Answer from the drawing. Dimensions are ordinates in mm from the lowest x, y and z of the part. A direction names the side the tool comes from. Give positions to 0.01 mm unless a question says otherwise; leave off trailing zeros. Order: outer loops, then holes, each group sorted by start corner. A loop starts at its lowest first (then second) coordinate and runs counter-clockwise, first axis right, second up.
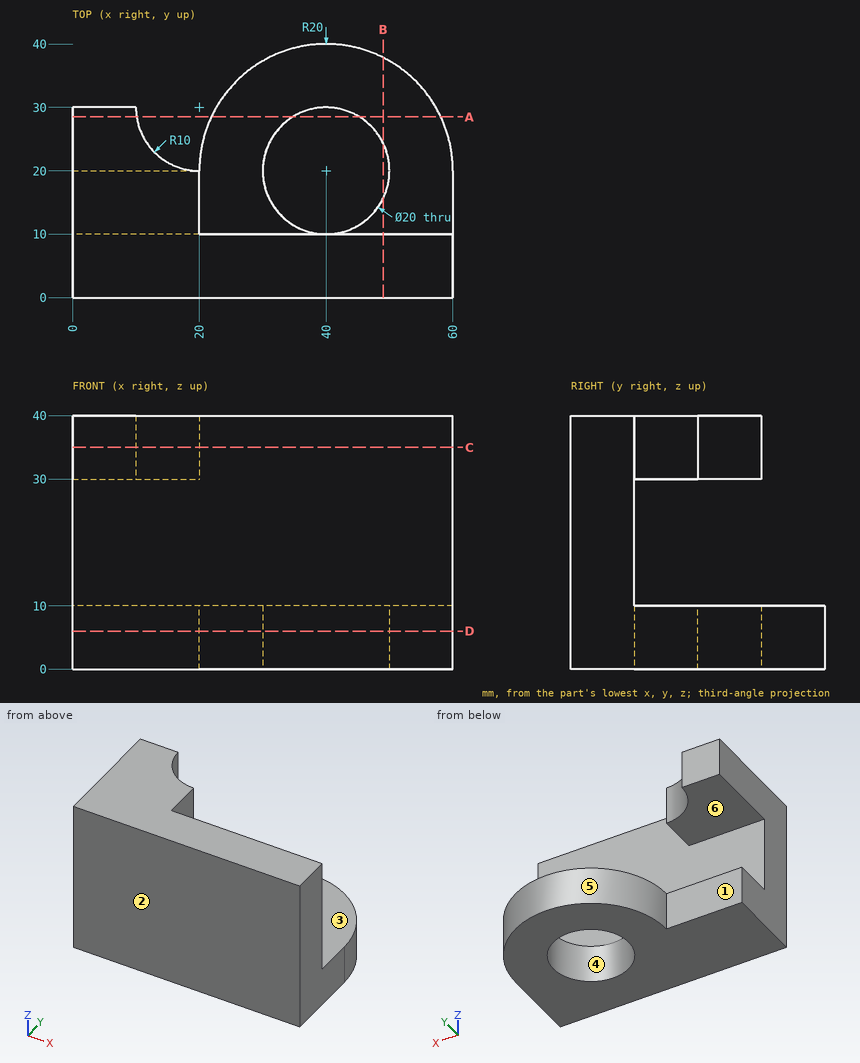
1. Given P1, Ø5, axis at x = 46, z = 26.5, coming from the -Y side; P2, Ø15, axis at x = 22.5, z = 21.5, coming from the +Y side; P3, Ø3, axis at x = 4.5, z = 34, coming from the +Y side; P4, Ø3, axis at y = 15.5, z = 32.5, coming from the +X side, each flat-ended and moving along its own axis, determine where each tip first touches the part or whether it passes through.
Findings below:
P1: stops at y = 0
P2: stops at y = 10
P3: stops at y = 30
P4: stops at x = 20
2. The part is cut by section C-C (z = 35). Write down the section's boundary in (x, y), then the cut area to 3 significant figures.
Findings below:
outline: (0, 0) - (60, 0) - (60, 10) - (20, 10) - (20, 20) arc R10 cw to (10, 30) - (0, 30) - close
area: 921 mm2
3. Straight lines are drawn through the part: probe 1 along Z at (x, y) = (19, 17); probe 2 along Z at (x, y) = (22, 20). For each, find the intervals that lie inside material, in ascending order.
Findings below:
probe 1: z = 0 to 10, 30 to 40
probe 2: z = 0 to 10
4. The part is cut by section A-A (y = 28.5). Write down the section's boundary in (x, z), then the cut area to 3 significant figures.
Findings below:
outline: (0, 30) - (10.11, 30) - (10.11, 40) - (0, 40) - close; (21.9, 0) - (34.73, 0) - (34.73, 10) - (21.9, 10) - close; (45.27, 0) - (58.1, 0) - (58.1, 10) - (45.27, 10) - close
area: 358 mm2
5. Which of the six approach directions +Z, -Z, +X, -X, +Y, -Y give full straight-line access (tool end or side, diameter ignored) to the marked faces 1, 2 and 3?
Findings below:
face 1: -Z, -X, +Y
face 2: +Z, -Z, +X, -X, -Y
face 3: +X, -X, +Y
6. The mould has two halves that part along X. Classify the marked faces 4, 5 and 6: pulls with the +X half, pulls with the -X half, needs draft (parallel to the pull), parting line crosses it, or undercut.
Findings below:
face 4: undercut
face 5: parting line crosses it
face 6: needs draft
7. The part is cut by section D-D (z = 6). Write down the section's boundary in (x, y).
Findings below:
outline: (0, 0) - (60, 0) - (60, 20) arc R20 ccw to (20, 20) - (0, 20) - close; hole circle Ø20 at (40, 20)
8. The part is cut by section B-B (x = 49). Write down the section's boundary in (y, z).
Findings below:
outline: (0, 0) - (15.64, 0) - (15.64, 10) - (10, 10) - (10, 40) - (0, 40) - close; (24.36, 0) - (37.86, 0) - (37.86, 10) - (24.36, 10) - close
